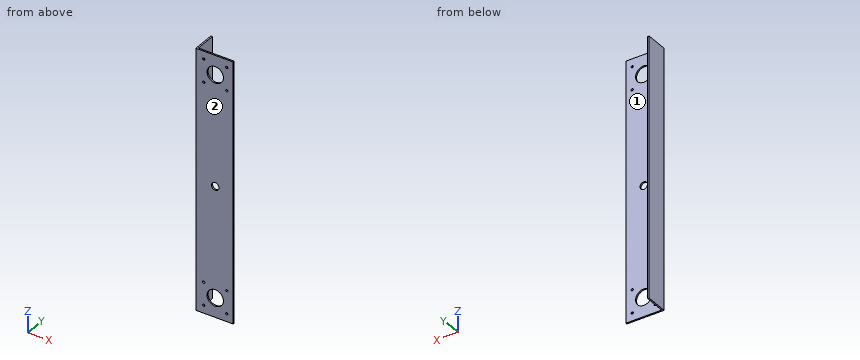
```python
from build123d import *

# Parameters (mm, degrees)
BOSS_EXTRUDE1_DEPTH = 350
SKETCH6_R           = 1.5
CUT_EXTRUDE3_DEPTH  = 355.660400947
SKETCH7_R           = 11
CUT_EXTRUDE4_DEPTH  = 355.660400947
SKETCH8_R           = 11
CUT_EXTRUDE5_DEPTH  = 355.823899984
SKETCH9_R           = 1.5
CUT_EXTRUDE6_DEPTH  = 355.823899984
SKETCH10_R          = 5
CUT_EXTRUDE7_DEPTH  = 355.823899984


with BuildPart() as part:
    # Sketch1 → Boss-Extrude1 (new body)
    with BuildSketch(Plane.XY):
        Polygon((0, 0), (0, 30), (2, 30), (2, 2), (50, 2), (50, 0), align=None)
    extrude(amount=BOSS_EXTRUDE1_DEPTH)

    # Sketch6 → Cut-Extrude3 (cut, through all)
    with BuildSketch(Plane(origin=(0, 2, 0), x_dir=(1, 0, 0), z_dir=(0, 1, 0))):
        with Locations(Location((41.5, -339.5, 0), (0, 0, 270))):
            Circle(SKETCH6_R)
        with Locations(Location((10.5, -308.5, 0), (0, 0, 270))):
            Circle(SKETCH6_R)
        with Locations(Location((10.5, -339.5, 0), (0, 0, 270))):
            Circle(SKETCH6_R)
        with Locations(Location((41.5, -308.5, 0), (0, 0, 270))):
            Circle(SKETCH6_R)
    extrude(amount=-CUT_EXTRUDE3_DEPTH, mode=Mode.SUBTRACT)

    # Sketch7 → Cut-Extrude4 (cut, through all)
    with BuildSketch(Plane(origin=(0, 2, 0), x_dir=(1, 0, 0), z_dir=(0, 1, 0))):
        with Locations(Location((26, -324, 0), (0, 0, 270))):
            Circle(SKETCH7_R)
    extrude(amount=-CUT_EXTRUDE4_DEPTH, mode=Mode.SUBTRACT)

    # Sketch8 → Cut-Extrude5 (cut, through all)
    with BuildSketch(Plane(origin=(0, 0, 0), x_dir=(-1, 0, 0), z_dir=(0, -1, 0))):
        with Locations(Location((-26, -26, 0), (0, 0, 180))):
            Circle(SKETCH8_R)
    extrude(amount=-CUT_EXTRUDE5_DEPTH, mode=Mode.SUBTRACT)

    # Sketch9 → Cut-Extrude6 (cut, through all)
    with BuildSketch(Plane.XZ):
        with Locations((41.5, 41.5)):
            Circle(SKETCH9_R)
        with Locations((10.5, 41.5)):
            Circle(SKETCH9_R)
        with Locations((10.5, 10.5)):
            Circle(SKETCH9_R)
        with Locations((41.5, 10.5)):
            Circle(SKETCH9_R)
    extrude(amount=-CUT_EXTRUDE6_DEPTH, mode=Mode.SUBTRACT)

    # Sketch10 → Cut-Extrude7 (cut, through all)
    with BuildSketch(Plane.XZ):
        with Locations((26.000000572, 175)):
            Circle(SKETCH10_R)
    extrude(amount=-CUT_EXTRUDE7_DEPTH, mode=Mode.SUBTRACT)


solid = part.part
```
Source: CAD feature listing. Evaluate the final solid. Frame: model axes, mm. Face numbers are marked on the shaded views. A direction names the side the tool comes from. Coordinates: 2 decimals unless noted, no trailing zeros. Loops run counter-clockwise (first coordinate to the right, second up) from the corner with the lowest first, then second, coordinate; pieces in that order, holes last. Notation, with made-up numbers: M 80,4 L 86,4 A19 cw 86,13 Z; hole C 77,-18 d4. An arc over 180 degrees is marked long. Put each result on its own line as item: value. Start each with the question number.
1) Cut plane A-A on z = 175. Return the cut outline in (x, y).
2) Cut plane C-C on z = 300.5. Return the cut outline in (x, y), then the cut area to 3 significant figures.
3) Ray query, L1, parallel to X at y = 0.75, z = 339.5; L2, parallel to Y at x = 12, z = 270.5. Return the intervals inside material, ascending. Write a range as from..to.
4) Cut plane D-D on y = 9.75. Return the cut outline in (x, z).
5) Contact query for flat-ended pins moving along their axis: pin 1 Ø1 at (x, z) = (44, 167.5) entering from +Y; pin 2 Ø2.5 at (x, z) = (41.5, 10.5) entering from +Y; pin 3 Ø10 at (y, z) = (20, 282) entering from -X; pin 4 Ø8.5 at (y, z) = (19, 211) entering from +X. Output: stop coordinate, or through.
6) Cut plane B-B on x = 26. Return the cut outline in (y, z), then the cut area to 3 significant figures.
7) Reachability of the marked faces 1 and 2 from +Z, -Z, +X, -X, +Y, -Y: full face, straight path, thin tool, end or side. Return the list, or none.
The answers:
1. outline: M 0,0 L 21,0 L 21,2 L 2,2 L 2,30 L 0,30 Z; M 31,0 L 50,0 L 50,2 L 31,2 Z
2. outline: M 0,0 L 50,0 L 50,2 L 2,2 L 2,30 L 0,30 Z
2. area: 156 mm²
3. L1: x = 0..9, 12..40, 43..50
3. L2: y = 0..2
4. outline: M 0,0 L 2,0 L 2,350 L 0,350 Z
5. pin 1: stops at y = 2
5. pin 2: passes through
5. pin 3: stops at x = 0
5. pin 4: stops at x = 2
6. outline: M 0,0 L 2,0 L 2,15 L 0,15 Z; M 0,37 L 2,37 L 2,170 L 0,170 Z; M 0,180 L 2,180 L 2,313 L 0,313 Z; M 0,335 L 2,335 L 2,350 L 0,350 Z
6. area: 592 mm²
7. face 1: +Z, -Z, +X, +Y
7. face 2: +Z, -Z, +X, -X, -Y
